```python
from build123d import *

# Parameters (mm, degrees)
EXTRUDE_THIN1_DEPTH = 609.6
EXTRUDE_THIN3_DEPTH = 609.6


with BuildPart() as part:
    # Sketch1 → Extrude-Thin1 (new body)
    with BuildSketch(Plane(origin=(0, 0, 0), x_dir=(1, 0, 0), z_dir=(0, 1, 0))):
        with BuildLine():
            Line((-863.6, 152.4), (863.6, 152.4))
            ThreePointArc((863.6, 152.4), (899.521024484, 137.521024484), (914.4, 101.6))
            Line((914.4, 101.6), (914.4, -101.6))
            ThreePointArc((914.4, -101.6), (899.521024484, -137.521024484), (863.6, -152.4))
            Line((863.6, -152.4), (-863.6, -152.4))
            ThreePointArc((-863.6, -152.4), (-899.521024484, -137.521024484), (-914.4, -101.6))
            Line((-914.4, -101.6), (-914.4, 101.6))
            ThreePointArc((-914.4, 101.6), (-899.521024484, 137.521024484), (-863.6, 152.4))
        make_face()
        with BuildLine():
            Line((-863.6, 130.175), (863.6, 130.175))
            ThreePointArc((863.6, 130.175), (883.805576272, 121.805576272), (892.175, 101.6))
            Line((892.175, 101.6), (892.175, -101.6))
            ThreePointArc((892.175, -101.6), (883.805576272, -121.805576272), (863.6, -130.175))
            Line((863.6, -130.175), (-863.6, -130.175))
            ThreePointArc((-863.6, -130.175), (-883.805576272, -121.805576272), (-892.175, -101.6))
            Line((-892.175, -101.6), (-892.175, 101.6))
            ThreePointArc((-892.175, 101.6), (-883.805576272, 121.805576272), (-863.6, 130.175))
        make_face(mode=Mode.SUBTRACT)
    extrude(amount=EXTRUDE_THIN1_DEPTH)

    # Sketch2 → Extrude-Thin3 (add)
    with BuildSketch(Plane(origin=(0, 609.6, 0), x_dir=(1, 0, 0), z_dir=(0, 1, 0))):
        Polygon((-884.317275894, -138.032724106), (-631.825, 114.459551788), (-371.475, -145.890448212), (-111.125, 114.459551788), (149.225, -145.890448212), (409.575, 114.459551788), (670.56979597, -146.535244182), (900.626773031, 122.960071803), (883.723226969, 137.389928197), (669.28020403, -113.814755818), (409.575, 145.890448212), (149.225, -114.459551788), (-111.125, 145.890448212), (-371.475, -114.459551788), (-631.825, 145.890448212), (-900.032724106, -122.317275894), align=None)
    extrude(amount=-EXTRUDE_THIN3_DEPTH)


solid = part.part
```
Model file for the job. Use its own axes, mm. A direction names the side the tool comes from. Give positions to 0.01 mm unless a question says otherwise; leave off trailing zeros. Write each loop counter-clockwise with the first axis right and the second up, starting at its lowest first coordinate (ties: lowest second). Pieces come first, ordered by that corner, then holes. Notation, with made-up numbers: (88.25, 26) - (120.25, 26) arc R18 cw to (120.25, 61) - close; hole circle Ø10 at (75.5, 34.25). An arc over 180 degrees is marked (long way). One line per question, with ' | ' between items. Start each with the question number.
(1) 3-axis set-ups, long thin cutter, end or side, ignore diameter. For faces 1 (the face through (899.914, 300.533, 137.124)), 2 (the face through (-492.08, 309.067, -6.145)): which of +Z, -Z, +X, -X, +Y, -Y reach the whole face in a straight line?
(2) Two-plate mould, pull along X, no slides. Class faces 3 (the face through (-899.124, 300.533, 137.914)), 4 (the face through (899.124, 300.533, -137.914)), 5 (the face through (773.78, 309.07, -8.6)): +X half, -X half, draft (parallel to the pull), parting line (faces both ways), or undercut.
(3) Wall check: line 1 along Z through (x, y) = (-257.5, 112.5) (3 decimals); line 2 along Z through (x, y) = (83, 276.5) (3 decimals); line 3 along X through (y, z) = (487, -131). Give the ranges that are in metal, low to high. Write a range as from..to.
(4) Slice it at A-A on x = 804. Write the cut outline in (y, z) (3 decimals), plus the area to 3 significant figures.
(5) Slice it at C-C on x = -144.5. Write the cut outline in (y, z) (3 decimals), plus the area to 3 significant figures.
(6) Slice it at B-B on y = 408. Give the number of separate pieces and of enclosed holes in the cut face, plus the area to 3 significant figures.
Results below:
1) face 1: +Z, +X, +Y, -Y | face 2: +Y, -Y
2) face 3: -X half | face 4: +X half | face 5: undercut
3) line 1: -152.4..-130.175, 0.485..31.915, 130.175..152.4 | line 2: -152.4..-130.175, 48.235..79.665, 130.175..152.4 | line 3: -905.03..905.03
4) outline: (0, -152.4) - (609.6, -152.4) - (609.6, -130.175) - (0, -130.175) - close; (0, -44) - (609.6, -44) - (609.6, -9.769) - (0, -9.769) - close; (0, 130.175) - (609.6, 130.175) - (609.6, 152.4) - (0, 152.4) - close | area: 48,000 mm^2
5) outline: (0, -152.4) - (609.6, -152.4) - (609.6, -130.175) - (0, -130.175) - close; (0, -112.515) - (609.6, -112.515) - (609.6, -81.085) - (0, -81.085) - close; (0, 130.175) - (609.6, 130.175) - (609.6, 152.4) - (0, 152.4) - close | area: 46,300 mm^2
6) separate pieces: 1 | enclosed holes: 8 | area: 146,000 mm^2
